```python
from build123d import *

# Parameters (mm, degrees)
ESQUISSE4_R             = 1.05
ENL_V_MAT_EXTRU_1_DEPTH = 32.032241298
ESQUISSE5_R             = 1.55
ENL_V_MAT_EXTRU_2_DEPTH = 31.757112998


with BuildPart() as part:
    # Esquisse3 → Révolution2 (revolve)
    with BuildSketch(Plane.XY):
        Polygon((-21, 23.3897956), (-21, 20.3897956), (-14, 20.3897956), (-14, 12.3897956), (-4.25, 12.3897956), (-4.25, 14.3897956), (-11, 14.3897956), (-11, 23.3897956), align=None)
    revolve(axis=Axis((0, 36.82979074, 0), (0, -1, 0)))

    # Esquisse4 → Enlèv. mat.-Extru.1 (cut, through all)
    with BuildSketch(Plane(origin=(0, 14.3897956, 0), x_dir=(1, 0, 0), z_dir=(0, 1, 0))):
        with Locations(Location((0, 8, 0), (0, 0, 180))):
            Circle(ESQUISSE4_R)
        with Locations(Location((5.656854249, 5.656854249, 0), (0, 0, 180))):
            Circle(ESQUISSE4_R)
        with Locations(Location((8, 0, 0), (0, 0, 180))):
            Circle(ESQUISSE4_R)
        with Locations(Location((5.656854249, -5.656854249, 0), (0, 0, 180))):
            Circle(ESQUISSE4_R)
        with Locations(Location((0, -8, 0), (0, 0, 180))):
            Circle(ESQUISSE4_R)
        with Locations(Location((-5.656854249, -5.656854249, 0), (0, 0, 180))):
            Circle(ESQUISSE4_R)
        with Locations(Location((-8, 0, 0), (0, 0, 180))):
            Circle(ESQUISSE4_R)
        with Locations(Location((-5.656854249, 5.656854249, 0), (0, 0, 180))):
            Circle(ESQUISSE4_R)
    extrude(amount=-ENL_V_MAT_EXTRU_1_DEPTH, mode=Mode.SUBTRACT)

    # Esquisse5 → Enlèv. mat.-Extru.2 (cut, through all)
    with BuildSketch(Plane.XZ.offset(-20.3897956)):
        with Locations((0, 17.05)):
            Circle(ESQUISSE5_R)
        with Locations((17.05, 0)):
            Circle(ESQUISSE5_R)
        with Locations((0, -17.05)):
            Circle(ESQUISSE5_R)
        with Locations((-17.05, 0)):
            Circle(ESQUISSE5_R)
    extrude(amount=-ENL_V_MAT_EXTRU_2_DEPTH, mode=Mode.SUBTRACT)


solid = part.part
```
The listing builds one solid part. Answer for the finished solid, in the listing's coordinates (mm). A direction names the side the tool comes from. Give positions to 0.01 mm unless a question says otherwise; leave off trailing zeros. Order: outer loops, then holes, each group sorted by start corner. A loop starts at its lowest first (then second) coordinate and runs counter-clockwise, first axis right, second up. Notation, with made-up numbers: (55, 37) - (109, 37) arc R13 ccw to (109, 62) - close; hole circle Ø3 at (21.25, 44). An arc over 180 degrees is marked (long way). Answer in a Markdown table with one row per item. Add a question column.
Q1. Which of the six approach directions +Z, -Z, +X, -X, +Y, -Y give full straight-line access (tool end or side, diameter ignored) to faces 4 (the flat face through (5, 14.39, 0)), 5 (the cylindrical face through (0.715, 21.869, -18.425))?
Q2. The part is cut by section C-C (z = 18). Determine the outline of the cut face in (x, y).
Q3. For a pull along Z with two mould halves and no side action, classify faces 1 (the cylindrical face through (-12.932, 16.334, 5.362)), 2 (the cylindrical face through (-18.6, 21.87, 0.07)), 3 (the flat face through (0.3, 20.39, -14.3)) as released by +Z, released by -Z, zero draft, split by the parting line, or undercut.
Q4. Find the intervals of material crossed by line 1 along Z through (x, y) = (0, 13.5); line 2 along Z through (x, y) = (-0.5, 14.5); line 3 along X through (y, z) = (13.5, 5), in increasing order. Write a range as [from, to].
Q5. The part is cut by section A-A (x = 0). Give the number of separate pieces and of enclosed holes in the cut face, then the cut area to 3 significant figures.
Q6. Given P1, Ø2, axis at x = -1, y = 19.5, coming from the -Z side; P2, Ø2, axis at y = 14.5, z = 2, coming from the -X side; P3, Ø5, axis at x = -17.05, z = 0, coming from the -Y side, each flat-ended and moving along its own axis, determine where each tip first touches the part or whether it passes through.
Determined:
| question | item | result |
|---|---|---|
| 1 | face 4 | +Y |
| 1 | face 5 | +Y, -Y |
| 2 | outline | (-10.82, 20.39) - (-1.22, 20.39) - (-1.22, 23.39) - (-10.82, 23.39) - close; (1.22, 20.39) - (10.82, 20.39) - (10.82, 23.39) - (1.22, 23.39) - close |
| 3 | face 1 | split by the parting line |
| 3 | face 2 | undercut |
| 3 | face 3 | zero draft |
| 4 | line 1 | z = [-14, -9.05], [-6.95, -4.25], [4.25, 6.95], [9.05, 14] |
| 4 | line 2 | z = [-13.99, -10.99], [10.99, 13.99] |
| 4 | line 3 | x = [-13.08, -6.48], [-4.84, 4.84], [6.48, 13.08] |
| 5 | separate pieces | 6 |
| 5 | enclosed holes | 0 |
| 5 | area | 108 mm² |
| 6 | P1 | stops at z = -20.99 |
| 6 | P2 | stops at x = -13.96 |
| 6 | P3 | stops at y = 20.39 |
